The figure shows three views and two pictorial views of one solid part (mm, origin at its lowest corner). Answer the questions. Give positions to 0.01 mm unless a question says otherwise; leave off trailing zeros. Loops run counter-clockwise (first coordinate to the right, second up) from the corner with the lowest first, then second, coordinate; pieces in that order, holes last. Notation, with made-up numbers: M 59.5,1.5 L 68.5,1.5 A22 cw 68.5,30.5 Z; hole C 0,42.5 d2. An arc over 180 degrees is marked long. One line per item, written item: value. Start each with the question number.
Q1. A cutting plane is placed at C-C, the plane y = 16.75. Determine the outline of the cut face in (x, z).
Q2. A cutting plane is placed at A-A, the plane z = 0.8. Determine the outline of the cut face in (x, y) (1 decimal), and give its area (3 significant figures).
Q3. Consider L1, parallel to Y at x = 5.25, z = 0.35 (1 decimal); L2, parallel to Y at x = 3.75, z = 0.2 (1 decimal); L3, parallel to X at y = 15.5, z = 0.6 (1 decimal). Determine where each line is inside the solid, lowest interval first.
Q4. A cutting plane is placed at B-B, the plane x = 20.75. Determine the outline of the cut face in (y, z), and give its area (3 significant figures).
Q5. The mould has two halves that part along X. Classify the marked faces 1 and 2: +X half, -X half, draft (parallel to the pull), parting line (faces both ways), or undercut.
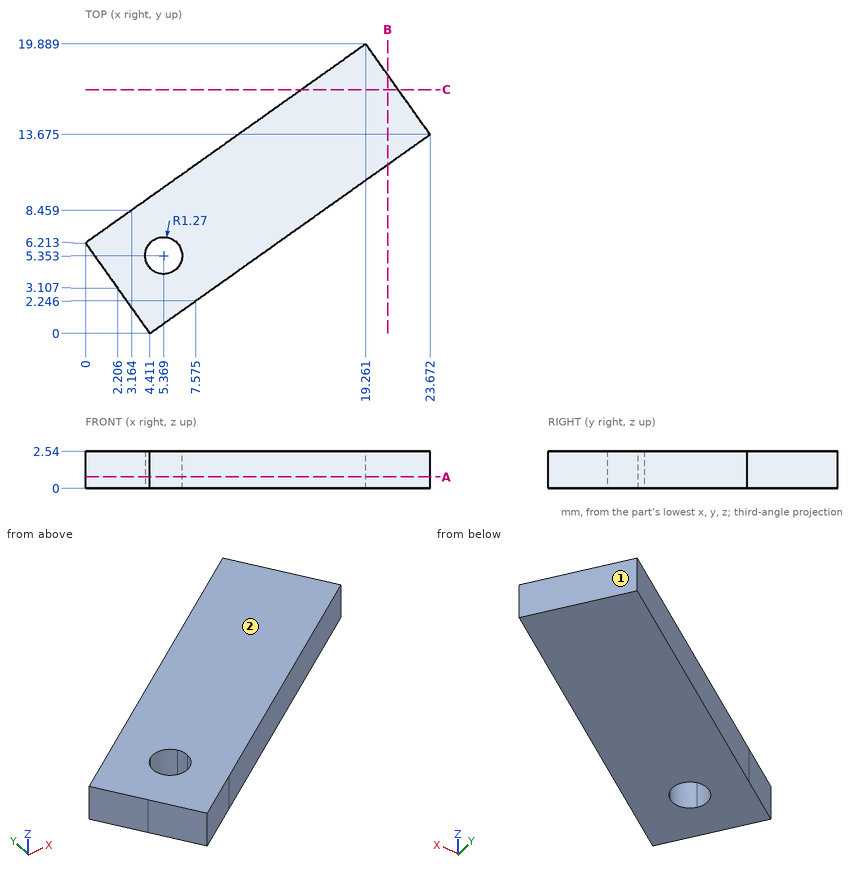
Answer block:
1. outline: M 14.84,0 L 21.49,0 L 21.49,2.54 L 14.84,2.54 Z
2. outline: M 0,6.2 L 4.4,0 L 23.7,13.7 L 19.3,19.9 Z; hole C 5.4,5.4 d2.5
2. area: 175 mm^2
3. L1: 0.6 to 4.1, 6.6 to 9.9
3. L2: 0.9 to 8.9
3. L3: 13.1 to 22.4
4. outline: M 11.6,0 L 17.79,0 L 17.79,2.54 L 11.6,2.54 Z
4. area: 15.7 mm^2
5. face 1: +X half
5. face 2: draft
